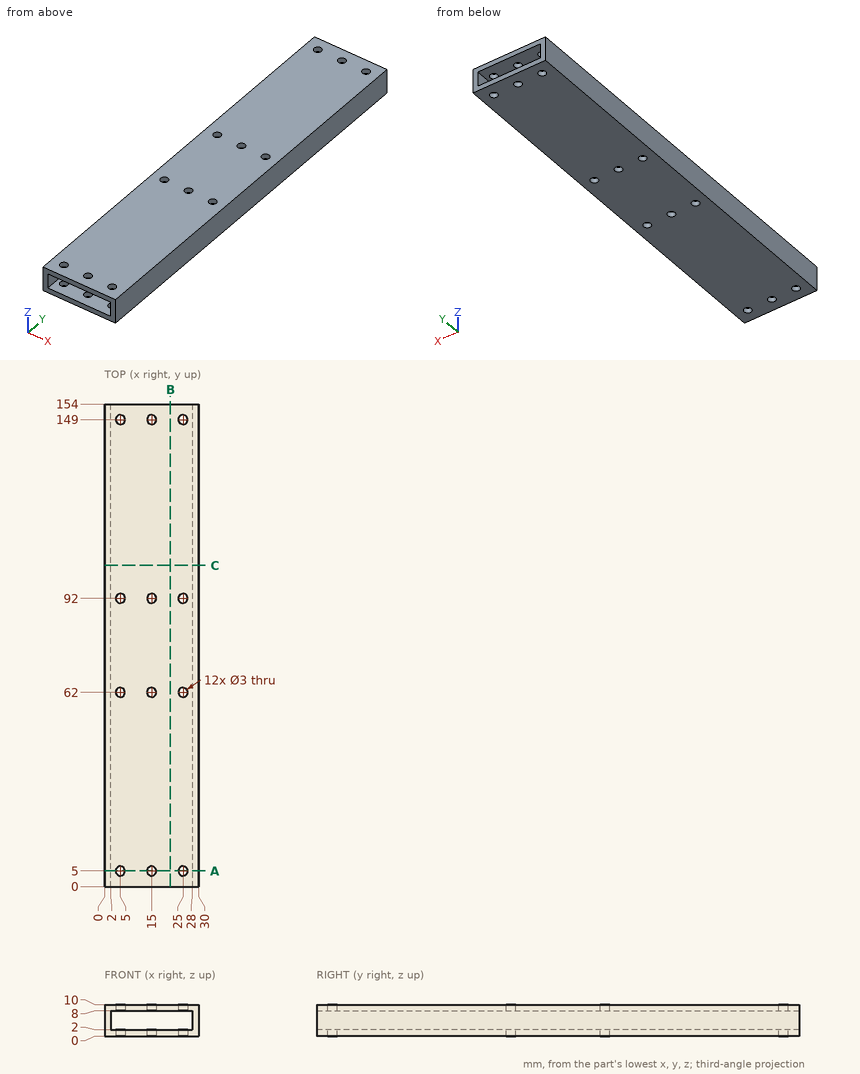
Print and shaded views of the part. All mm, measured from the part's lowest x, y and z. Round coordinates to 2 decimals unless told otherwise and drop trailing zeros. Loops run counter-clockwise (first coordinate to the right, second up) from the corner with the lowest first, then second, coordinate; pieces in that order, holes last. Notation, with made-up numbers: (87.25, -33) -> (125.25, -33) arc R15 cw to (125.25, -6) -> close; hole circle Ø8 at (-6, 53). An arc over 180 degrees is marked (long way). Use CSV: the item, a comma, the result in double quotes. Start each with the question number.
1) Cut at B-B, the plane x = 21. Write the cut outline in (y, z).
2) Cut at A-A, the plane y = 5. Give the number of separate pieces and of enclosed holes in the cut face, plus the area to 3 significant figures.
3) Wall check: L1, parallel to X at y = 92, z = 0.6; L2, parallel to Y at x = 15, z = 9.25; L3, parallel to X at y = 87, z = 2.75. Give the ranges that are in metal, low to high. Write a range as [from, to].
4) Cut at C-C, the plane y = 102.5. Write the cut outline in (x, z), plus the area to 3 significant figures.
5) Drop a flat-ended pin along its axis: P1, Ø1.5, axis at x = 25.5, z = 7, coming from the +Y side. Give the stop position or say it passes through.
Determined:
1,outline,"(0, 0) -> (154, 0) -> (154, 2) -> (0, 2) -> close; (0, 8) -> (154, 8) -> (154, 10) -> (0, 10) -> close"
2,separate pieces,"6"
2,enclosed holes,"0"
2,area,"108 mm2"
3,L1,"x = [0, 3.5], [6.5, 13.5], [16.5, 23.5], [26.5, 30]"
3,L2,"y = [0, 3.5], [6.5, 60.5], [63.5, 90.5], [93.5, 147.5], [150.5, 154]"
3,L3,"x = [0, 2], [28, 30]"
4,outline,"(0, 0) -> (30, 0) -> (30, 10) -> (0, 10) -> close; hole (2, 2) -> (28, 2) -> (28, 8) -> (2, 8) -> close"
4,area,"144 mm2"
5,P1,"passes through"
